```python
from build123d import *

# Parameters (mm, degrees)
SKETCH1_R           = 4
BOSS_EXTRUDE1_DEPTH = 30
FILLET1_R           = 10
CUT_EXTRUDE1_DEPTH  = 50


with BuildPart() as part:
    # Sketch1 → Boss-Extrude1 (new body)
    with BuildSketch(Plane.XY):
        with BuildLine():
            Line((138.386569071, 266.427133764), (138.503487168, 271.253231947))
            ThreePointArc((138.503487168, 271.253231947), (132.941191098, 289.393266743), (126.507007076, 271.543861264))
            Line((126.507007076, 271.543861264), (126.433420754, 268.506394661))
            ThreePointArc((126.433420754, 268.506394661), (124.910300495, 265.601515317), (122.784429578, 263.103737869))
            ThreePointArc((122.784429578, 263.103737869), (43.666158034, 141.541101292), (29.413949453, -2.798948778))
            ThreePointArc((29.413949453, -2.798948778), (38.103150753, -19.665773564), (41.273132032, -0.959004301))
            ThreePointArc((41.273132032, -0.959004301), (55.014402731, 137.639339628), (131.004003349, 254.360820334))
            ThreePointArc((131.004003349, 254.360820334), (135.506043856, 259.89792897), (138.386569071, 266.427133764))
        make_face()
        with Locations((36.57, -9.784)):
            Circle(SKETCH1_R, mode=Mode.SUBTRACT)
        with Locations((132.699, 279.3962)):
            Circle(SKETCH1_R, mode=Mode.SUBTRACT)
    extrude(amount=-BOSS_EXTRUDE1_DEPTH)

    # Fillet1
    fillet1_edges = [part.edges().sort_by_distance(p)[0] for p in [
        (41.273132032, -0.959004301, -15),
        (29.413949453, -2.798948778, -15),
    ]]
    fillet(fillet1_edges, radius=FILLET1_R)

    # Sketch2 → Cut-Extrude1 (cut, symmetric)
    with BuildSketch(Plane(origin=(35.859794138, -11.920477788, 0), x_dir=(0, 0, -1), z_dir=(0.948943265, -0.315446794, 0))):
        with BuildLine():
            Line((18, -41.651017654), (18, 72.25142837))
            ThreePointArc((18, 72.25142837), (17.213593845, 86.688920515), (14.863680684, 100.955578225))
            ThreePointArc((14.863680684, 100.955578225), (3.726945122, 168.568287043), (0, 236.990616386))
            Line((0, 236.990616386), (-79.914214629, -10.518807221))
            Line((-79.914214629, -10.518807221), (18, -41.651017654))
        make_face()
        with BuildLine():
            ThreePointArc((12, 236.990616386), (15.655931666, 169.871851405), (26.580467348, 103.547278514))
            ThreePointArc((26.580467348, 103.547278514), (29.14258039, 87.992484876), (30, 72.25142837))
            Line((30, 72.25142837), (155.717662302, 285.460245478))
            Line((155.717662302, 285.460245478), (12, 328.230650316))
            Line((12, 328.230650316), (12, 236.990616386))
        make_face()
    extrude(amount=CUT_EXTRUDE1_DEPTH, both=True, mode=Mode.SUBTRACT)


solid = part.part
```
Verification items for the finished model (mm, model axes). A direction names the side the tool comes from. Coordinates: 2 decimals unless noted, no trailing zeros. Write each loop counter-clockwise with the first axis right and the second up, starting at its lowest first coordinate (ties: lowest second). Pieces come first, ordered by that corner, then holes. Notation, with made-up numbers: M 57.25,22.25 L 80.25,22.25 A22 cw 80.25,52.25 Z; hole C 38.25,2 d5. An arc over 180 degrees is marked long. Answer as a JSON object with one key per item and string values. Group by question number.
(1) Gauge pin test, flat ends, axial feed: pin 1 (6 mm diameter, centred on y = 36.5, z = -19, fed in from +X); pin 2 (10.5 mm diameter, centred on x = 36.57, y = -9.784, fed in from +Z); pin 3 (8 mm diameter, centred on x = 69.5, z = -15, fed in from +Y); pin 4 (10.5 mm diameter, centred on x = 132.7, y = 279.4, fed in from +Z). Record the tip position at first contact, or that the pin passes through.
(2) Material ranges on line 1 (Y direction, x = 96.5, z = -7); line 2 (X direction, y = 191.5, z = -7.5); line 3 (X direction, y = 262.5, z = -5), recorded low to high.
(3) Tool access check on faces 5 (the face through (55.062, 137.776, -14.79)), 6 (the face through (124.936, 265.64, -5.916)). Record the directions out of +Z, -Z, +X, -X, +Y, -Y that give a thin tool (end or side, any length) a straight path to the whole face; none if there is none.
(4) Cross-section at A-A, the plane y = 26. Record the cut outline in (x, z), and give its area (3 significant figures).
(5) Release check for a two-part mould opening along Y. For faces 1 (the face through (135.45, 259.81, -5.92)), 2 (the face through (133.29, 289.38, -5.92)), 3 (the face through (37.73, -19.717, -23.916)), 4 (the face through (34, 23, -18)) record: +Y half, -Y half, draft (parallel to the pull), parting line (faces both ways), or undercut.
Reply:
{
 "1": {"pin 1": "x = 38.46", "pin 2": "z = -18", "pin 3": "y = 201.79", "pin 4": "z = 0"},
 "2": {"line 1": "215.64 to 235.08", "line 2": "66.43 to 80.33", "line 3": "122.14 to 136.91"},
 "3": {"face 5": "+Z, -Z, +X", "face 6": "+Z, -Z, -X"},
 "4": {"outline": "M 26.71,-30 L 38.72,-30 L 38.72,-18 L 26.71,-18 Z", "area": "144 mm²"},
 "5": {"face 1": "-Y half", "face 2": "undercut", "face 3": "undercut", "face 4": "draft"}
}
